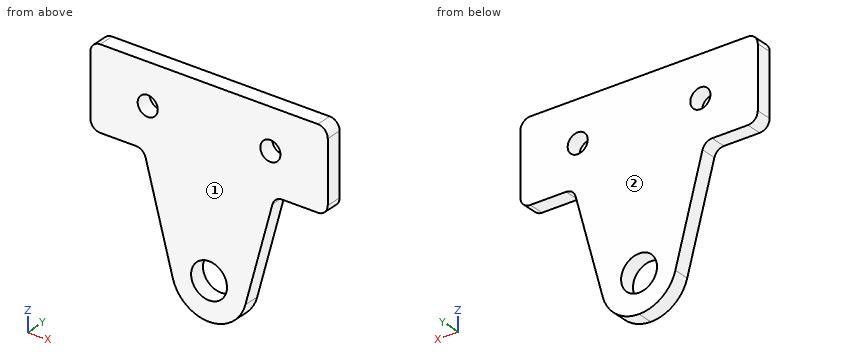
from build123d import *
from build123d import SkipClean  # not in build123d's __all__

# Parameters (mm, degrees)
F0_R     = 5.075
F1_DEPTH = 8


with BuildPart() as f1:
    # F0 (on Front) → F1 (new body)
    with BuildSketch(Plane.XZ):
        with BuildLine():
            ThreePointArc((-18.3525906995, 14.0824381431), (-11.5664671512, 3.9262865345), (0, 0))
            Line((0, 0), (0, 9.925))
            ThreePointArc((0, 9.925), (-9.075, 19), (0, 28.075))
            Line((0, 28.075), (0, 110))
            Line((0, 110), (-55, 110))
            ThreePointArc((-55, 110), (-58.5355339059, 108.5355339059), (-60, 105))
            Line((-60, 105), (-60, 74))
            ThreePointArc((-60, 74), (-58.5355339059, 70.4644660941), (-55, 69))
            Line((-55, 69), (-36.9043419892, 69))
            ThreePointArc((-36.9043419892, 69), (-33.8605348442, 67.9667667015), (-32.0747128578, 65.2940952255))
            Line((-32.0747128578, 65.2940952255), (-18.3525906995, 14.0824381431))
        make_face()
        with Locations((-31, 89.5)):
            Circle(F0_R, mode=Mode.SUBTRACT)
    extrude(amount=F1_DEPTH)

    # F2: F1 across face


with BuildPart() as f1_1:
    add(f1.part, clean=False)
    with SkipClean():  # cleaning this boolean's faces spoils the solid; the shape is the same uncleaned
        add(f1.part.mirror(Plane(origin=(0, -4, 69.0375), x_dir=(0, 1, 0), z_dir=(1, 0, 0))), clean=False)


solid = f1_1.part
The listing builds one solid part. Answer for the finished solid, in the listing's coordinates (mm). Face numbers are marked on the shaded views. Give positions to 0.01 mm unless a question says otherwise; leave off trailing zeros. Write each loop counter-clockwise with the first axis right and the second up, starting at its lowest first coordinate (ties: lowest second). Pieces come first, ordered by that corner, then holes. Notation, with made-up numbers: (-29.75, 49.5) - (27.25, 49.5) arc R25 cw to (27.25, 83.5) - close; hole circle Ø2 at (68, 23.25). An arc over 180 degrees is marked (long way). Use a Markdown table: item, result.
1. This flat-tipped pin is pushed along its axis until it touches: P1, Ø9, axis at x = 31, z = 89.5, coming from the -Y side. Where does it stop, or does it pass through?
Values follow:
| item | result |
|---|---|
| P1 | passes through |
2. Section B-B on y = -5.25 is taken. Write down the section's boundary in (x, z) (3 decimals).
Values follow:
| item | result |
|---|---|
| outline | (-60, 74) arc R5 ccw to (-55, 69) - (-36.904, 69) arc R5 cw to (-32.075, 65.294) - (-18.353, 14.082) arc R19 ccw to (18.353, 14.082) - (32.075, 65.294) arc R5 cw to (36.904, 69) - (55, 69) arc R5 ccw to (60, 74) - (60, 105) arc R5 ccw to (55, 110) - (-55, 110) arc R5 ccw to (-60, 105) - close; hole circle Ø10.15 at (-31, 89.5); hole circle Ø18.15 at (0, 19); hole circle Ø10.15 at (31, 89.5) |
3. Section D-D on x = -44.5 is taken. Write down the section's boundary in (y, z), plus the area to 3 significant figures.
Values follow:
| item | result |
|---|---|
| outline | (-8, 69) - (0, 69) - (0, 110) - (-8, 110) - close |
| area | 328 mm² |
4. Section A-A on z = 89.5 is taken. Write down the section's boundary in (x, y) (3 decimals), plus the area to 3 significant figures.
Values follow:
| item | result |
|---|---|
| outline | (-60, -8) - (-36.075, -8) - (-36.075, 0) - (-60, 0) - close; (-25.925, -8) - (25.925, -8) - (25.925, 0) - (-25.925, 0) - close; (36.075, -8) - (60, -8) - (60, 0) - (36.075, 0) - close |
| area | 798 mm² |
5. For a pull along Y with two mould halves and no side action, classify the marked faces 1 and 2 as released by +Y, released by -Y, zero draft, split by the parting line, or undercut.
Values follow:
| item | result |
|---|---|
| face 1 | released by -Y |
| face 2 | released by +Y |
6. Find the intervals of material crossed by probe 1 along X at (y, z) = (-1.5, 90); probe 2 along Z at (x, y) = (0, -5.25) (3 decimals); probe 3 along Z at (x, y) = (53.5, -1.25), in increasing order. Write a range as from..to.
Values follow:
| item | result |
|---|---|
| probe 1 | x = -60..-36.05, -25.95..25.95, 36.05..60 |
| probe 2 | z = 0..9.925, 28.075..110 |
| probe 3 | z = 69..110 |
7. Section C-C on z = 19 is taken. Write down the section's boundary in (x, y) (3 decimals).
Values follow:
| item | result |
|---|---|
| outline | (-19.67, -8) - (-9.075, -8) - (-9.075, 0) - (-19.67, 0) - close; (9.075, -8) - (19.67, -8) - (19.67, 0) - (9.075, 0) - close |
